Geometry: final body of the model. Coordinates: model frame, mm. A direction names the side the tool comes from. Give positions to 0.01 mm unless a question says otherwise; leave off trailing zeros. Loops run counter-clockwise (first coordinate to the right, second up) from the corner with the lowest first, then second, coordinate; pieces in that order, holes last. Notation, with made-up numbers: M 73,-28.75 L 124,-28.75 A28 cw 124,-5.75 Z; hole C -35,46 d4. An arc over 180 degrees is marked long. Put each result on its own line as item: value.
```python
from build123d import *

# Parameters (mm, degrees)
SKETCH1_W                  = 72
SKETCH1_H                  = 13
SKETCH1_W_2                = 90
SKETCH1_H_2                = 40
BOSS_EXTRUDE1_DEPTH        = 6.5
FILLET2_R                  = 30
SKETCH2_R                  = 15
SKETCH2_R_2                = 1.6
MOTOR_CLEARANCE_DEPTH      = 105.648220243
CUT_SIDE_WHEEL_HOLES_REACH = 106.648
SKETCH3_W                  = 10
SKETCH3_H                  = 6.5
CUT_EXTRUDE1_REACH         = 106.648
SKETCH5_W                  = 20
SKETCH5_H                  = 6.5


with BuildPart() as part:
    # Sketch1 → Boss-Extrude1 (new body)
    with BuildSketch(Plane.XY):
        with Locations((45, 46.5)):
            Rectangle(SKETCH1_W, SKETCH1_H)
        with Locations((45, 20)):
            Rectangle(SKETCH1_W_2, SKETCH1_H_2)
    extrude(amount=BOSS_EXTRUDE1_DEPTH)

    # Fillet2
    fillet2_edges = [part.edges().sort_by_distance(p)[0] for p in [
        (90, 0, 3.25),
        (0, 0, 3.25),
    ]]
    fillet(fillet2_edges, radius=FILLET2_R)

    # Sketch2 → motor clearance (cut, through all)
    with BuildSketch(Plane.XY.offset(6.5)):
        with Locations((45, 52.639320225)):
            Circle(SKETCH2_R)
        with Locations((62.960512242, 52.639320225)):
            Circle(SKETCH2_R_2)
        with Locations((45, 34.678807983)):
            Circle(SKETCH2_R_2)
        with Locations((27.039487758, 52.639320225)):
            Circle(SKETCH2_R_2)
    extrude(amount=-MOTOR_CLEARANCE_DEPTH, mode=Mode.SUBTRACT)

    # Sketch3 → cut side wheel holes (cut, up to next)
    with BuildSketch(Plane.XY.offset(6.5), mode=Mode.PRIVATE) as cut_side_wheel_holes_sk1:
        with Locations((24, 43.25)):
            Rectangle(SKETCH3_W, SKETCH3_H)
    cut_side_wheel_holes_tool1 = extrude(cut_side_wheel_holes_sk1.sketch, amount=-CUT_SIDE_WHEEL_HOLES_REACH, mode=Mode.PRIVATE) & part.part
    # Sketch3 → cut side wheel holes (cut, up to next)
    with BuildSketch(Plane.XY.offset(6.5), mode=Mode.PRIVATE) as cut_side_wheel_holes_sk2:
        with Locations((66, 43.25)):
            Rectangle(SKETCH3_W, SKETCH3_H)
    cut_side_wheel_holes_tool2 = extrude(cut_side_wheel_holes_sk2.sketch, amount=-CUT_SIDE_WHEEL_HOLES_REACH, mode=Mode.PRIVATE) & part.part
    add(cut_side_wheel_holes_tool1.solids().sort_by_distance((24, 43.25, 6.5))[0], mode=Mode.SUBTRACT)
    add(cut_side_wheel_holes_tool2.solids().sort_by_distance((66, 43.25, 6.5))[0], mode=Mode.SUBTRACT)

    # Sketch5 → Cut-Extrude1 (cut, up to next)
    with BuildSketch(Plane.XY.offset(6.5), mode=Mode.PRIVATE) as cut_extrude1_sk1:
        with Locations((45, 22.75)):
            Rectangle(SKETCH5_W, SKETCH5_H)
    cut_extrude1_tool1 = extrude(cut_extrude1_sk1.sketch, amount=-CUT_EXTRUDE1_REACH, mode=Mode.PRIVATE) & part.part
    # Sketch5 → Cut-Extrude1 (cut, up to next)
    with BuildSketch(Plane.XY.offset(6.5), mode=Mode.PRIVATE) as cut_extrude1_sk2:
        with Locations((45, 9.75)):
            Rectangle(SKETCH5_W, SKETCH5_H)
    cut_extrude1_tool2 = extrude(cut_extrude1_sk2.sketch, amount=-CUT_EXTRUDE1_REACH, mode=Mode.PRIVATE) & part.part
    add(cut_extrude1_tool1.solids().sort_by_distance((45, 22.75, 6.5))[0], mode=Mode.SUBTRACT)
    add(cut_extrude1_tool2.solids().sort_by_distance((45, 9.75, 6.5))[0], mode=Mode.SUBTRACT)


solid = part.part
```
Item 1: Set-up query: faces 1 (the flat face through (90, 35, 3)), 2 (the flat face through (35, 10, 3)), 3 (the flat face through (4, 40, 3)). Return all of +Z, -Z, +X, -X, +Y, -Y with unobstructed straight access to the full face (end or side cutting, diameter ignored); none if empty.
Output values:
face 1: +Z, -Z, +X, +Y, -Y
face 2: +Z, -Z
face 3: +Z, -Z, -X, +Y
Item 2: Pin query (flat end, axial travel): pin 1 Ø2 at (x, z) = (9, 1.5) entering from -Y; pin 2 Ø3 at (y, z) = (11, 4.5) entering from +X; pin 3 Ø2 at (x, z) = (43.5, 3) entering from +Y. Return the tip coordinate at first contact, or that it passes through.
Output values:
pin 1: y = 7.64
pin 2: x = 84.37
pin 3: y = 37.85
Item 3: Line query: probe 1 along Y at (x, z) = (45, 3); probe 2 along Y at (x, z) = (38, 3.5); probe 3 along Y at (x, z) = (50, 1). Output: solid intervals per line, ascending. Write a range as [from, to].
Output values:
probe 1: [0, 6.5], [13, 19.5], [26, 33.08], [36.28, 37.64]
probe 2: [0, 6.5], [13, 19.5], [26, 39.37]
probe 3: [0, 6.5], [13, 19.5], [26, 38.5]
Item 4: Mould query, pull axis Y, two halves, no side actions, for faces 4 (the cylindrical face through (80.979, 8.555, 3.296)), 5 (the flat face through (85, 40, 3)), 6 (the flat face through (61, 43, 3)), 7 (the flat face through (19, 43, 3)). Classes: pulls with the +Y half, pulls with the -Y half, needs draft (parallel to the pull), parting line crosses it, or undercut.
Output values:
face 4: pulls with the -Y half
face 5: pulls with the +Y half
face 6: undercut
face 7: undercut
Item 5: Section B-B on y = 20.5. Output: boundary loops of the cut face in (x, z), then the cut area to 3 significant figures.
Output values:
outline: M 1.54,0 L 35,0 L 35,6.5 L 1.54,6.5 Z; M 55,0 L 88.46,0 L 88.46,6.5 L 55,6.5 Z
area: 435 mm²
Item 6: Section D-D on x = 76. Output: boundary loops of the cut face in (y, z).
Output values:
outline: M 4.62,0 L 53,0 L 53,6.5 L 4.62,6.5 Z
Item 7: Section C-C on z = 3.25. Count the separate pieces of the cut face and the enclosed holes in it, then the cut area to 3 significant figures.
Output values:
separate pieces: 1
enclosed holes: 5
area: 3,380 mm²
Item 8: Section A-A on x = 45. Output: boundary loops of the cut face in (y, z), then the cut area to 3 significant figures.
Output values:
outline: M 0,0 L 6.5,0 L 6.5,6.5 L 0,6.5 Z; M 13,0 L 19.5,0 L 19.5,6.5 L 13,6.5 Z; M 26,0 L 33.08,0 L 33.08,6.5 L 26,6.5 Z; M 36.28,0 L 37.64,0 L 37.64,6.5 L 36.28,6.5 Z
area: 139 mm²
